CAD build for the part. Positions are in the model's coordinates, mm. A direction names the side the tool comes from. Round coordinates to 2 decimals unless told otherwise and drop trailing zeros. Order: outer loops, then holes, each group sorted by start corner. A loop starts at its lowest first (then second) coordinate and runs counter-clockwise, first axis right, second up. Notation, with made-up numbers: M 40,-30 L 81,-30 A8 ccw 81,-18 Z; hole C 69,-19.75 d2. An arc over 180 degrees is marked long. Answer as a JSON object with one key per item and string values.
```python
from build123d import *

# Parameters (mm, degrees)
SKETCH1_W           = 40.5
SKETCH1_H           = 76
BOSS_EXTRUDE1_DEPTH = 19
SKETCH2_R           = 13
BOSS_EXTRUDE2_DEPTH = 35
SKETCH3_W           = 48
SKETCH3_H           = 25.5
BOSS_EXTRUDE3_DEPTH = 30
SKETCH4_R           = 4.5
BOSS_EXTRUDE4_DEPTH = 5


with BuildPart() as part:
    # Sketch1 → Boss-Extrude1 (new, symmetric)
    with BuildSketch(Plane(origin=(0, 0, 0), x_dir=(0, 0, -1), z_dir=(1, 0, 0))):
        Rectangle(SKETCH1_W, SKETCH1_H)
    extrude(amount=BOSS_EXTRUDE1_DEPTH, both=True)

    # Sketch2 → Boss-Extrude2 (add)
    with BuildSketch(Plane.XZ.offset(38)):
        with Locations(Location((0, 0, 0), (0, 0, 270))):
            Circle(SKETCH2_R)
    extrude(amount=BOSS_EXTRUDE2_DEPTH)

    # Sketch3 → Boss-Extrude3 (add)
    with BuildSketch(Plane(origin=(0, 0, -15.25), x_dir=(-1, 0, 0), z_dir=(0, 0, -1))):
        with Locations((5, 50.75)):
            Rectangle(SKETCH3_W, SKETCH3_H)
    extrude(amount=-BOSS_EXTRUDE3_DEPTH)

    # Sketch4 → Boss-Extrude4 (add)
    with BuildSketch(Plane.ZY.offset(29)):
        with Locations(Location((0, 53.5, 0), (0, 0, 270))):
            Circle(SKETCH4_R)
    extrude(amount=BOSS_EXTRUDE4_DEPTH)


solid = part.part
```
Item 1: Saw through at D-D on x = -15. List the corners of the cut face in (y, z), and give its area (3 significant figures).
Worked answers:
{"outline": "M -38,-20.25 L 38,-20.25 L 38,-15.25 L 63.5,-15.25 L 63.5,14.75 L 38,14.75 L 38,20.25 L -38,20.25 Z", "area": "3,840 mm2"}
Item 2: 3-axis set-ups, long thin cutter, end or side, ignore diameter. For faces 5 (the flat face through (0, 38, 18)), 6 (the flat face through (0, 38, -18)), 7 (the flat face through (-24, 38, 0)): which of +Z, -Z, +X, -X, +Y, -Y reach the whole face in a straight line?
Worked answers:
{"face 5": "+Z, +X, -X, +Y", "face 6": "-Z, +X, -X, +Y", "face 7": "+Z, -Z, -X, -Y"}
Item 3: Two-plate mould, pull along X, no slides. Class faces 1 (the cylindrical face through (-7.91, -55.255, 10.316)), 2 (the flat face through (19, 12, 0)), 3 (the flat face through (-34, 54, 0)), 4 (the flat face through (13, -38, 5)): released by +X, released by -X, zero draft, split by the parting line, or undercut.
Worked answers:
{"face 1": "split by the parting line", "face 2": "released by +X", "face 3": "released by -X", "face 4": "zero draft"}
Item 4: Wall check: line 1 along X through (y, z) = (-34, 14); line 2 along Y through (x, z) = (-14.5, -14.5); line 3 along X through (y, z) = (58, -6). Give the ranges that are in metal, low to high. Write a range as [from, to].
Worked answers:
{"line 1": "x = [-19, 19]", "line 2": "y = [-38, 63.5]", "line 3": "x = [-29, 19]"}
Item 5: Saw through at B-B on y = 53.5. List the corners of the cut face in (x, z).
Worked answers:
{"outline": "M -34,-4.5 L -29,-4.5 L -29,-15.25 L 19,-15.25 L 19,14.75 L -29,14.75 L -29,4.5 L -34,4.5 Z"}
Item 6: Drop flat-ended pins along their axis: pin 1 Ø10 at (y, z) = (42, -13) entering from -X; pin 2 Ø5 at (x, z) = (-28, 2) entering from -Y; pin 3 Ø12 at (y, z) = (16, 8) entering from -X. Give the stop position or say it passes through.
Worked answers:
{"pin 1": "stops at x = -29", "pin 2": "stops at y = 38", "pin 3": "stops at x = -19"}
Item 7: Saw through at C-C on x = 5. List the corners of the cut face in (y, z).
Worked answers:
{"outline": "M -73,-12 L -38,-12 L -38,-20.25 L 38,-20.25 L 38,-15.25 L 63.5,-15.25 L 63.5,14.75 L 38,14.75 L 38,20.25 L -38,20.25 L -38,12 L -73,12 Z"}
Item 8: Saw through at A-A on z = 0. List the corners of the cut face in (x, y), and give its area (3 significant figures).
Worked answers:
{"outline": "M -34,49 L -29,49 L -29,38 L -19,38 L -19,-38 L -13,-38 L -13,-73 L 13,-73 L 13,-38 L 19,-38 L 19,63.5 L -29,63.5 L -29,58 L -34,58 Z", "area": "5,070 mm2"}
